from build123d import *

# Parameters (mm, degrees)
F0_R     = 50
F1_DEPTH = 10
F2_R     = 4.99999
F3_W     = 9.3445703387
F3_H     = 114.5939677954
F3_W_2   = 10.3282090276
F3_H_2   = 115.5776083469
F3_W_3   = 9.3445708044
F3_H_3   = 117.5448857248
F3_H_4   = 117.0530617237
F4_DEPTH = 1


# Not quite as in the source:
# - a fillet or chamfer is up to 0.001 mm smaller than in the source, because OpenCascade refuses the exact size


with BuildPart() as f1:
    # F0 (on Top) → F1 (new body)
    with BuildSketch(Plane.XY):
        Circle(F0_R)
    extrude(amount=F1_DEPTH)

    # F2 (radius 5 in the source; OpenCascade refuses exactly that, so slightly less here)
    f2_edges = [f1.edges().sort_by_distance(p)[0] for p in [
        (-50, 0, 0),
        (-50, 0, 10),
    ]]
    fillet(f2_edges, radius=F2_R)

    # F3 (on face) → F4 (cut)
    with BuildSketch(Plane(origin=(0, 0, 0), x_dir=(1, 0, 0), z_dir=(0, 0, -1))):
        with Locations((-36.148738116, -1.2295395136)):
            Rectangle(F3_W, F3_H)
        with Locations((-12.5413937494, -1.7213597894)):
            Rectangle(F3_W_2, F3_H_2)
        with Locations((11.5577613469, -2.2131819278)):
            Rectangle(F3_W_3, F3_H_3)
        with Locations((32.7060082927, -2.9509104788)):
            Rectangle(F3_W_2, F3_H_4)
    extrude(amount=-F4_DEPTH, mode=Mode.SUBTRACT)


solid = f1.part
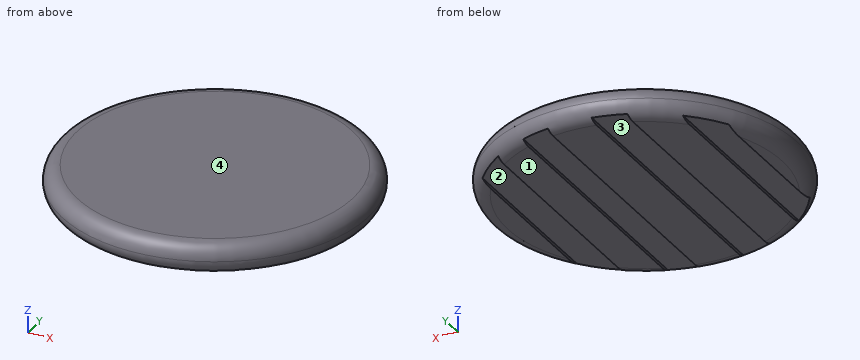
Geometry: final body of the model. Coordinates: model frame, mm. Face numbers are marked on the shaded views. A direction names the side the tool comes from. Give positions to 0.01 mm unless a question says otherwise; leave off trailing zeros. Return JSON: item names as keys, results as strings. Group by question number.
1) Mould query, pull axis X, two halves, no side actions, for the marked faces 1 and 2. Classes: released by +X, released by -X, zero draft, split by the parting line, or undercut.
2) Line query: line 1 (X direction, y = -22, z = 0.5); line 2 (Z direction, x = 13.5, y = -40); line 3 (Y direction, x = 26, z = 5.25). Output: solid intervals per line, ascending.
3) Set-up query: the marked faces 3 and 4. Return all of +Z, -Z, +X, -X, +Y, -Y with unobstructed straight access to the full face (end or side cutting, diameter ignored); none if empty.
4) First-contact query: P1, Ø4, axis at y = 33, z = 4, coming from the -X side; P2, Ø1.1, axis at y = -8, z = 0.5, coming from the +X side; P3, Ø3, axis at x = -13, y = -14.5, coming from the -Z side. Flat tips, straight axial feed; report the tip coordinate or a pass-through.
Filled in:
{
 "1": {"face 1": "zero draft", "face 2": "undercut"},
 "2": {"line 1": "x = -41.74 to -40.82, -31.48 to -17.71, -7.38 to 6.89, 16.23 to 27.54, 37.87 to 41.74", "line 2": "z = 1 to 10", "line 3": "y = -42.7 to 42.7"},
 "3": {"face 3": "-Z, +Y, -Y", "face 4": "+Z, +X, -X, +Y, -Y"},
 "4": {"P1": "stops at x = -39.15", "P2": "stops at x = 47.4", "P3": "stops at z = 1"}
}
